Verification items for the finished model (mm, model axes). Coordinates: 2 decimals unless noted, no trailing zeros. Order: outer loops, then holes, each group sorted by start corner. A loop starts at its lowest first (then second) coordinate and runs counter-clockwise, first axis right, second up. Notation, with made-up numbers: M 22.25,17 L 39.25,17 A35 ccw 39.25,53 Z; hole C 9.5,20.25 d4. An arc over 180 degrees is marked long. Return JSON: item names as keys, results as strings. Group by question number.
Q1. Section check D-D, the plane x = 44. Enter the section's corners in (y, z) (3 decimals), then the cut area to 3 significant figures.
Q2. Mould release check, pull along Z, two halves, no side actions. Record for faces 1 (the face through (39.265, -3.131, -10.346)), 2 (the face through (63.5, -3, -1)), 3 (the face through (-1, -3, -47.625)), 4 (the face through (-1, -3, 47.625)): pulls with the +Z half, pulls with the -Z half, needs draft (parallel to the pull), parting line crosses it, or undercut.
Q3. Section check A-A, the plane x = -36.83. Count the separate pieces of the cut face and the enclosed holes in it, then the cut area to 3 significant figures.
Q4. Go/stop test with a flat-tipped pin: pin 1 Ø4.5 at (x, z) = (-36.83, -11.11) entering from -Y. Record where the tip stops, or that it passes through.
Q5. Thickness scan on probe 1 along Z at (x, y) = (36.83, -4.25) (1 decimal); probe 2 along Z at (x, y) = (0, -4.5) (3 decimals); probe 3 along X at (y, z) = (-1.5, 7). Record the ranges inside material, lowest first.
Q6. Section check B-B, the plane x = 0. Enter the section's corners in (y, z) (3 decimals).
from build123d import *

# Parameters (mm, degrees)
F0_W     = 127
F0_H     = 95.25
F0_R     = 2.5527
F0_R_2   = 14.2875
F0_R_3   = 11.43
F0_R_4   = 11.1125
F1_DEPTH = 6.35


with BuildPart() as f1:
    # F0 (on Front) → F1 (new body)
    with BuildSketch(Plane.XZ):
        Rectangle(F0_W, F0_H)
        with Locations((-36.83, -11.1125)):
            Circle(F0_R, mode=Mode.SUBTRACT)
        with Locations((0, -21.2725)):
            Circle(F0_R_2, mode=Mode.SUBTRACT)
        with Locations((36.83, -11.1125)):
            Circle(F0_R, mode=Mode.SUBTRACT)
        with Locations((-36.83, 14.2875)):
            Circle(F0_R_3, mode=Mode.SUBTRACT)
        with Locations((-36.83, 39.6875)):
            Circle(F0_R, mode=Mode.SUBTRACT)
        with Locations((0, 14.2875)):
            Circle(F0_R_4, mode=Mode.SUBTRACT)
        with Locations((36.83, 14.2875)):
            Circle(F0_R_3, mode=Mode.SUBTRACT)
        with Locations((36.83, 39.6875)):
            Circle(F0_R, mode=Mode.SUBTRACT)
    extrude(amount=F1_DEPTH)


solid = f1.part
Numbers:
{
 "1": {"outline": "M -6.35,-47.625 L 0,-47.625 L 0,5.386 L -6.35,5.386 Z; M -6.35,23.189 L 0,23.189 L 0,47.625 L -6.35,47.625 Z", "area": "492 mm2"},
 "2": {"face 1": "undercut", "face 2": "needs draft", "face 3": "pulls with the -Z half", "face 4": "pulls with the +Z half"},
 "3": {"separate pieces": "4", "enclosed holes": "0", "area": "395 mm2"},
 "4": {"pin 1": "passes through"},
 "5": {"probe 1": "z = -47.6 to -13.7, -8.6 to 2.9, 25.7 to 37.1, 42.2 to 47.6", "probe 2": "z = -47.625 to -35.56, -6.985 to 3.175, 25.4 to 47.625", "probe 3": "x = -63.5 to -45.64, -28.02 to -8.39, 8.39 to 28.02, 45.64 to 63.5"},
 "6": {"outline": "M -6.35,-47.625 L 0,-47.625 L 0,-35.56 L -6.35,-35.56 Z; M -6.35,-6.985 L 0,-6.985 L 0,3.175 L -6.35,3.175 Z; M -6.35,25.4 L 0,25.4 L 0,47.625 L -6.35,47.625 Z"}
}
